Part model, mm, in its own coordinate system. A direction names the side the tool comes from. Coordinates: 2 decimals unless noted, no trailing zeros. Order: outer loops, then holes, each group sorted by start corner. A loop starts at its lowest first (then second) coordinate and runs counter-clockwise, first axis right, second up.
from build123d import *

# Parameters (mm, degrees)
SKETCH_R     = 4.76
PAD_DEPTH    = 6.35
SKETCH001_R  = 6.35
PAD001_DEPTH = 26.2
SKETCH002_R  = 1
PAD002_DEPTH = 11.7
SKETCH003_R  = 2.5
PAD003_DEPTH = 11
PAD004_DEPTH = 2
FILLET_R     = 1


with BuildPart() as part:
    # Sketch → Pad (new body)
    with BuildSketch(Plane.XY):
        Circle(SKETCH_R)
    extrude(amount=PAD_DEPTH)

    # Sketch001 (on Face3 of Pad) → Pad001 (join)
    with BuildSketch(Plane.XY.offset(6.35)):
        Circle(SKETCH001_R)
    extrude(amount=PAD001_DEPTH)

    # Sketch002 (on Face5 of Pad001) → Pad002 (join)
    with BuildSketch(Plane(origin=(0, 0, 0), x_dir=(1, 0, 0), z_dir=(0, 0, -1))):
        Circle(SKETCH002_R)
    extrude(amount=PAD002_DEPTH)

    # Sketch003 (on Face3 of Pad002) → Pad003 (join)
    with BuildSketch(Plane.XY.offset(32.55)):
        Circle(SKETCH003_R)
    extrude(amount=PAD003_DEPTH)

    # Sketch004 (on Face3 of Pad003) → Pad004 (join)
    with BuildSketch(Plane.XY.offset(32.55)):
        with BuildLine():
            ThreePointArc((1.736759, 5.586248), (0, 5.85), (-1.736759, 5.586248))
            Line((-1.736759, 4.421105), (-1.736759, 5.586248))
            ThreePointArc((1.736759, 4.421105), (0, 4.75), (-1.736759, 4.421105))
            Line((1.736759, 5.586248), (1.736759, 4.421105))
        make_face()
    extrude(amount=PAD004_DEPTH)

    # Fillet
    fillet_edges = [part.edges().sort_by_distance(p)[0] for p in [
        (-6.35, 0, 32.55),
    ]]
    fillet(fillet_edges, radius=FILLET_R)


solid = part.part
Q1. Mould opens along Y. For faces 5 (the face through (0.02, 5.85, 33.54)), 6 (the face through (0, 1, -6)), 7 (the face through (0.02, 4.75, 33.54)), 8 (the face through (-1, -5, 6.35)) say: pulls with the +Y half, pulls with the -Y half, needs draft (parallel to the pull), parting line crosses it, or undercut.
Results list:
face 5: pulls with the +Y half
face 6: parting line crosses it
face 7: undercut
face 8: needs draft
Q2. Wall check: line 1 along Y through (x, z) = (0, -2.5); line 2 along Z through (x, y) = (-2.25, -4.75); line 3 along Z through (x, y) = (2.5, -0.5). Give the ranges that are in metal, low to high.
Results list:
line 1: y = -1 to 1
line 2: z = 6.35 to 32.55
line 3: z = 0 to 32.55
Q3. Cut at B-B on z = 28.5. Write the cut outline in (x, y).
Results list:
outline: circle Ø12.7 at (0, 0)
Q4. Cut at C-C on z = 5. Write the cut outline in (x, y).
Results list:
outline: circle Ø9.52 at (0, 0)
Q5. Which spindle directions (+Z, -Z, +X, -X, +Y, -Y) get a long thin tool onto all of the face, cutting with end or side? Do faces 1 (the face through (-1.737, 5, 34)), 2 (the face through (1.737, 5, 34)), 3 (the face through (-0.54, -2.44, 37.97)), 4 (the face through (0, 5, 34.55)). Say none if no direction does.
Results list:
face 1: +Z, -X, +Y
face 2: +Z, +X, +Y
face 3: +Z
face 4: +Z, +X, -X, +Y
Q6. Pin check, flat tips, straight feed: pin 1 Ø4 at (y, z) = (4, 2) entering from +X; pin 2 Ø1.5 at (x, z) = (2, 20) entering from -Y; pin 3 Ø3 at (x, z) = (-1.5, 0) entering from +Y. Stop position of each tip, or through.
Results list:
pin 1: stops at x = 4.32
pin 2: stops at y = -6.23
pin 3: stops at y = 4.76
Q7. Cut at A-A on y = 0. Write the cut outline in (x, z).
Results list:
outline: (-6.35, 6.35) - (-4.76, 6.35) - (-4.76, 0) - (-1, 0) - (-1, -11.7) - (1, -11.7) - (1, 0) - (4.76, 0) - (4.76, 6.35) - (6.35, 6.35) - (6.35, 31.55) arc R1 ccw to (5.35, 32.55) - (2.5, 32.55) - (2.5, 43.55) - (-2.5, 43.55) - (-2.5, 32.55) - (-5.35, 32.55) arc R1 ccw to (-6.35, 31.55) - close
